```python
from build123d import *

# Parameters (mm, degrees)
ESQUISSE1_W                  = 140
ESQUISSE1_H                  = 140
ESQUISSE1_W_2                = 5
ESQUISSE1_H_2                = 20
BOSS_EXTRU_1_DEPTH           = 13.5
ENL_V_MAT_EXTRU_3_DEPTH      = 8.5
ENL_V_MAT_EXTRU_1_DEPTH      = 100
R_P_TITION_CIRCULAIRE1_COUNT = 2
R_P_TITION_CIRCULAIRE1_ANGLE = 90
CONG_1_R                     = 10
ESQUISSE3_R                  = 1.5
ENL_V_MAT_EXTRU_2_DEPTH      = 13.5


with BuildPart() as part:
    # Esquisse1 → Boss.-Extru.1 (new body)
    with BuildSketch(Plane(origin=(0, 0, 0), x_dir=(1, 0, 0), z_dir=(0, 1, 0))):
        Rectangle(ESQUISSE1_W, ESQUISSE1_H)
        with Locations((-27.5, 25)):
            Rectangle(ESQUISSE1_W_2, ESQUISSE1_H_2, mode=Mode.SUBTRACT)
        Polygon((65, 12.5), (55, 2.5), (55, 32.5), (65, 42.5), align=None, mode=Mode.SUBTRACT)
        Polygon((65, -12.5), (55, -2.5), (55, -32.5), (65, -42.5), align=None, mode=Mode.SUBTRACT)
        Polygon((12.5, -65), (2.5, -55), (32.5, -55), (42.5, -65), align=None, mode=Mode.SUBTRACT)
        Polygon((-12.5, -65), (-2.5, -55), (-32.5, -55), (-42.5, -65), align=None, mode=Mode.SUBTRACT)
        Polygon((-65, -12.5), (-55, -2.5), (-55, -32.5), (-65, -42.5), align=None, mode=Mode.SUBTRACT)
        Polygon((-65, 12.5), (-55, 2.5), (-55, 32.5), (-65, 42.5), align=None, mode=Mode.SUBTRACT)
        Polygon((-12.5, 65), (-2.5, 55), (-32.5, 55), (-42.5, 65), align=None, mode=Mode.SUBTRACT)
        Polygon((12.5, 65), (2.5, 55), (32.5, 55), (42.5, 65), align=None, mode=Mode.SUBTRACT)
        with Locations((-27.5, -15)):
            Rectangle(ESQUISSE1_W_2, ESQUISSE1_H_2, mode=Mode.SUBTRACT)
        with Locations((27.5, 25)):
            Rectangle(ESQUISSE1_W_2, ESQUISSE1_H_2, mode=Mode.SUBTRACT)
        with Locations((27.5, -15)):
            Rectangle(ESQUISSE1_W_2, ESQUISSE1_H_2, mode=Mode.SUBTRACT)
    extrude(amount=BOSS_EXTRU_1_DEPTH)

    # Esquisse4 → Enl_v. mat.-Extru.3 (cut)
    with BuildSketch(Plane(origin=(0, 13.5, 0), x_dir=(1, 0, 0), z_dir=(0, 1, 0))):
        Polygon((-21.715728753, -50), (21.715728753, -50), (50, -21.715728753), (50, 21.715728753), (21.715728753, 50), (-21.715728753, 50), (-50, 21.715728753), (-50, -21.715728753), align=None)
    extrude(amount=-ENL_V_MAT_EXTRU_3_DEPTH, mode=Mode.SUBTRACT)

    # Esquisse2 → Enl_v. mat.-Extru.1 (cut, symmetric)
    with BuildSketch(Plane(origin=(0, 0, 0), x_dir=(0.707106781, 0, -0.707106781), z_dir=(0.707106781, 0, 0.707106781))):
        with BuildLine():
            Line((-6, 14), (6, 14))
            ThreePointArc((6, 14), (0, 8), (-6, 14))
        make_face()
    enl_v_mat_extru_1 = extrude(amount=ENL_V_MAT_EXTRU_1_DEPTH, both=True, mode=Mode.SUBTRACT)

    # R_p_tition circulaire1: Enl_v. mat.-Extru.1 ×2 about axis
    r_p_tition_circulaire1_axis = Axis((0, -76.187687151, 0), (0, 1, 0))
    for i in range(1, R_P_TITION_CIRCULAIRE1_COUNT):
        add(enl_v_mat_extru_1.rotate(r_p_tition_circulaire1_axis, i * R_P_TITION_CIRCULAIRE1_ANGLE / (R_P_TITION_CIRCULAIRE1_COUNT - 1)), mode=Mode.SUBTRACT)

    # Cong_1
    cong_1_edges = [part.edges().sort_by_distance(p)[0] for p in [
        (-70, 4, -70),
        (-70, 4, 70),
        (70, 4, -70),
        (70, 4, 70),
        (21.715728753, 9.25, -50),
        (50, 9.25, -21.715728753),
        (50, 9.25, 21.715728753),
        (21.715728753, 9.25, 50),
        (-21.715728753, 9.25, 50),
        (-50, 9.25, 21.715728753),
        (-21.715728753, 9.25, -50),
        (-50, 9.25, -21.715728753),
    ]]
    fillet(cong_1_edges, radius=CONG_1_R)

    # Esquisse3 → Enl_v. mat.-Extru.2 (cut)
    with BuildSketch(Plane(origin=(0, 13.5, 0), x_dir=(-1, 0, 0), z_dir=(0, 1, 0))):
        with Locations((44.443650814, 60)):
            Circle(ESQUISSE3_R)
        with Locations((60, 44.443650814)):
            Circle(ESQUISSE3_R)
        with Locations((60, -44.443650814)):
            Circle(ESQUISSE3_R)
        with Locations((44.443650814, -60)):
            Circle(ESQUISSE3_R)
        with Locations((-44.443650814, -60)):
            Circle(ESQUISSE3_R)
        with Locations((-60, -44.443650814)):
            Circle(ESQUISSE3_R)
        with Locations((-60, 44.443650814)):
            Circle(ESQUISSE3_R)
        with Locations((-44.443650814, 60)):
            Circle(ESQUISSE3_R)
        with Locations((49.393398282, 33.837049096)):
            Circle(ESQUISSE3_R)
        with Locations((33.837049096, 49.393398282)):
            Circle(ESQUISSE3_R)
        with Locations((33.837049096, -49.393398282)):
            Circle(ESQUISSE3_R)
        with Locations((49.393398282, -33.837049096)):
            Circle(ESQUISSE3_R)
        with Locations((-49.393398282, -33.837049096)):
            Circle(ESQUISSE3_R)
        with Locations((-33.837049096, -49.393398282)):
            Circle(ESQUISSE3_R)
        with Locations((-33.837049096, 49.393398282)):
            Circle(ESQUISSE3_R)
        with Locations((-49.393398282, 33.837049096)):
            Circle(ESQUISSE3_R)
        with Locations((12.5, -12.5)):
            Circle(ESQUISSE3_R)
        with Locations((-12.5, -12.5)):
            Circle(ESQUISSE3_R)
        with Locations((-12.5, 12.5)):
            Circle(ESQUISSE3_R)
        with Locations((12.5, 12.5)):
            Circle(ESQUISSE3_R)
    extrude(amount=-ENL_V_MAT_EXTRU_2_DEPTH, mode=Mode.SUBTRACT)


solid = part.part
```
CAD build for the part. Positions are in the model's coordinates, mm. A direction names the side the tool comes from. Round coordinates to 2 decimals unless told otherwise and drop trailing zeros. Loops run counter-clockwise (first coordinate to the right, second up) from the corner with the lowest first, then second, coordinate; pieces in that order, holes last. Notation, with made-up numbers: M 30.5,22 L 79.5,22 A14 cw 79.5,33 Z; hole C 1.5,48.25 d8. An arc over 180 degrees is marked long. Return JSON: item names as keys, results as strings. Group by question number.
(1) Saw through at C-C, the plane x = -8. List the corners of the cut face in (y, z).
(2) Saw through at D-D, the plane y = 11.25. Give the number of separate pieces and of enclosed holes in the cut face, and give its area (3 significant figures).
(3) Saw through at A-A, the plane x = 6.5. List the corners of the cut face in (y, z).
(4) Tool access for faces 1 (the flat face through (-7.6, 6.7, 60.1)), 2 (the cylindrical face through (-49.26, 9.19, 21.35)): list every direction of +Z, -Z, +X, -X, +Y, -Y with a clear straight run to the whole face (end or side of a thin tool).
(5) Drop flat-ended pins along their axis: P1, Ø2.5, axis at x = 60, z = -44.44, coming from the -Y side; P2, Ø2, axis at x = 32, z = 11, coming from the +Y side. Give the stop position or say it passes through.
(6) Mould opens along Z. For faces 3 (the cylindrical face through (66.99, 5.34, 67.15)), 4 (the flat face through (-1, 13.5, -59)), 5 (the flat face through (-7.6, 6.7, -60.1)) say: +Z half, -Z half, draft (parallel to the pull), parting line (faces both ways), or undercut.
(7) Saw through at B-B, the plane z = -21. List the corners of the cut face in (x, y).
(8) Wall check: probe 1 along Z at (x, y) = (16.5, 13); probe 2 along Z at (x, y) = (-12.5, 1.4); probe 3 along Z at (x, y) = (-15, 1). Give the ranges that are in metal, low to high. Write a range as [from, to].
Answer list:
{
 "1": {"outline": "M 0,-70 L 13.5,-70 L 13.5,-60.5 L 0,-60.5 Z; M 0,-55 L 13.5,-55 L 13.5,-50 L 5,-50 L 5,50 L 13.5,50 L 13.5,55 L 0,55 Z; M 0,60.5 L 13.5,60.5 L 13.5,70 L 0,70 Z"},
 "2": {"separate pieces": "4", "enclosed holes": "24", "area": "6,760 mm2"},
 "3": {"outline": "M 0,-70 L 13.5,-70 L 13.5,-59 L 0,-59 Z; M 0,-55 L 13.5,-55 L 13.5,-50 L 5,-50 L 5,50 L 13.5,50 L 13.5,55 L 0,55 Z; M 0,59 L 13.5,59 L 13.5,70 L 0,70 Z"},
 "4": {"face 1": "+Y, -Y", "face 2": "+Y"},
 "5": {"P1": "through", "P2": "y = 5"},
 "6": {"face 3": "+Z half", "face 4": "draft", "face 5": "undercut"},
 "7": {"outline": "M -70,0 L -65,0 L -65,13.5 L -70,13.5 Z; M -55,0 L -30,0 L -30,5 L -49.39,5 L -49.39,13.5 L -55,13.5 Z; M -25,0 L 25,0 L 25,5 L -25,5 Z; M 30,0 L 55,0 L 55,13.5 L 49.39,13.5 L 49.39,5 L 30,5 Z; M 65,0 L 70,0 L 70,13.5 L 65,13.5 Z"},
 "8": {"probe 1": "[-70, -65], [-55, -50], [50, 55], [65, 70]", "probe 2": "[-70, -65], [-55, -14], [-11, 11], [14, 55], [65, 70]", "probe 3": "[-70, -65], [-55, 55], [65, 70]"}
}
